```python
from build123d import *

# Parameters (mm, degrees)
SKETCH1_R           = 69.85
SKETCH1_R_2         = 55.88
BOSS_EXTRUDE1_DEPTH = 3.175
SKETCH4_R           = 1.27
CUT_EXTRUDE2_DEPTH  = 108.317012813


with BuildPart() as part:
    # Sketch1 → Boss-Extrude1 (new body)
    with BuildSketch(Plane.XY):
        with Locations((-8.548720341, -3.365444156)):
            Circle(SKETCH1_R)
        with Locations((-8.548720341, -3.365444156)):
            Circle(SKETCH1_R_2, mode=Mode.SUBTRACT)
    extrude(amount=BOSS_EXTRUDE1_DEPTH)

    # Sketch4 → Cut-Extrude2 (cut, through all)
    with BuildSketch(Plane(origin=(0, 0, 0), x_dir=(-1, 0, 0), z_dir=(0, 0, -1))):
        with BuildLine():
            ThreePointArc((-28.926835269, 55.58033798), (-40.842688325, 46.02596451), (-50.397061795, 34.110111454))
            Line((-50.397061795, 34.110111454), (-34.971216033, 36.553325402))
            ThreePointArc((-34.971216033, 36.553325402), (-34.937133041, 36.590451286), (-34.903018379, 36.62754807))
            ThreePointArc((-34.903018379, 36.62754807), (-31.862432204, 37.045708389), (-31.444271885, 40.086294564))
            ThreePointArc((-31.444271885, 40.086294564), (-31.407175101, 40.120409226), (-31.370049217, 40.154492217))
            Line((-31.370049217, 40.154492217), (-28.926835269, 55.58033798))
        make_face()
        with BuildLine():
            ThreePointArc((46.024275952, -62.311226293), (57.940129007, -52.756852822), (67.494502478, -40.840999767))
            Line((67.494502478, -40.840999767), (52.068656715, -43.284213714))
            ThreePointArc((52.068656715, -43.284213714), (52.034573724, -43.321339599), (52.000459061, -43.358436383))
            ThreePointArc((52.000459061, -43.358436383), (48.959872886, -43.776596701), (48.541712568, -46.817182876))
            ThreePointArc((48.541712568, -46.817182876), (48.504615784, -46.851297539), (48.467489899, -46.88538053))
            Line((48.467489899, -46.88538053), (46.024275952, -62.311226293))
        make_face()
        with Locations((-50.506279659, -3.365444156)):
            Circle(SKETCH4_R)
        with Locations((8.548720341, -62.420444156)):
            Circle(SKETCH4_R)
        with Locations((8.548720341, 55.689555844)):
            Circle(SKETCH4_R)
        with Locations((67.603720341, -3.365444156)):
            Circle(SKETCH4_R)
    extrude(amount=-CUT_EXTRUDE2_DEPTH, mode=Mode.SUBTRACT)


solid = part.part
```
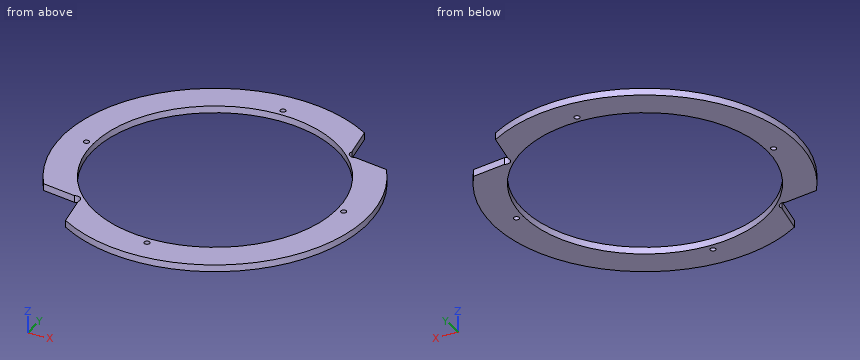
For this review, take the finished solid that the model builds, in its own axes (mm). Coordinates: 2 decimals unless noted, no trailing zeros. Loops run counter-clockwise (first coordinate to the right, second up) from the corner with the lowest first, then second, coordinate; pieces in that order, holes last. Notation, with made-up numbers: (-37, 13.25) - (-29, 13.25) arc R27 cw to (-29, 49.25) - close; hole circle Ø10 at (11, -7.5). An arc over 180 degrees is marked (long way). Use one line per item in the form item = value. Start each with the question number.
1) Take a section at B-B (y = -28). State the section outline as (x, z) points (1 decimal).
2) To check wall thickness, follow probe 1 along Y at (x, z) = (-9, 2.35); probe 2 along Y at (x, z) = (-26.5, 1.05); probe 3 along X at (y, z) = (-40, 2.8). State the ranges of each line that lie inside material, in increasing order. Write a range as from..to.
3) For pin 1 (3 mm diameter, centred on x = -67.6, y = -3.37, fed in from -Z), flat-tipped, find the tip position at first contact; note if it passes through.
4) Take a section at C-C (z = 1.6). State the section outline as (x, y) points, plus the area to 3 significant figures.
5) Take a section at A-A (x = 44). State the section outline as (y, z) points (3 decimals), plus the area to 3 significant figures.
From the geometry:
q1.outline = (-73.9, 0) - (-58.7, 0) - (-58.7, 3.2) - (-73.9, 3.2) - close; (41.6, 0) - (56.8, 0) - (56.8, 3.2) - (41.6, 3.2) - close
q2.probe_1 = -73.21..-63.61, -61.23..-59.24, 52.51..54.5, 56.88..66.48
q2.probe_2 = -70.87..-56.28, 49.55..64.14
q2.probe_3 = -68.02..-50.74, 33.65..50.92
q3.pin_1 = 0
q4.outline = (-67.49, -40.84) - (-52.07, -43.28) arc R59.05 ccw to (-52, -43.36) arc R2.54 cw to (-48.54, -46.82) arc R59.05 ccw to (-48.47, -46.89) - (-46.02, -62.31) arc R69.85 ccw to (50.4, 34.11) - (34.97, 36.55) arc R59.06 ccw to (34.9, 36.63) arc R2.54 cw to (31.44, 40.09) arc R59.06 ccw to (31.37, 40.15) - (28.93, 55.58) arc R69.85 ccw to start; hole circle Ø2.54 at (-67.6, -3.37); hole circle Ø111.76 at (-8.55, -3.37); hole circle Ø2.54 at (-8.55, -62.42); hole circle Ø2.54 at (-8.55, 55.69); hole circle Ø2.54 at (50.51, -3.37)
q4.area = 5,090 mm2
q5.outline = (-49.383, 0) - (-22.371, 0) - (-22.371, 3.175) - (-49.383, 3.175) - close; (15.64, 0) - (35.123, 0) - (35.123, 3.175) - (15.64, 3.175) - close
q5.area = 148 mm2
